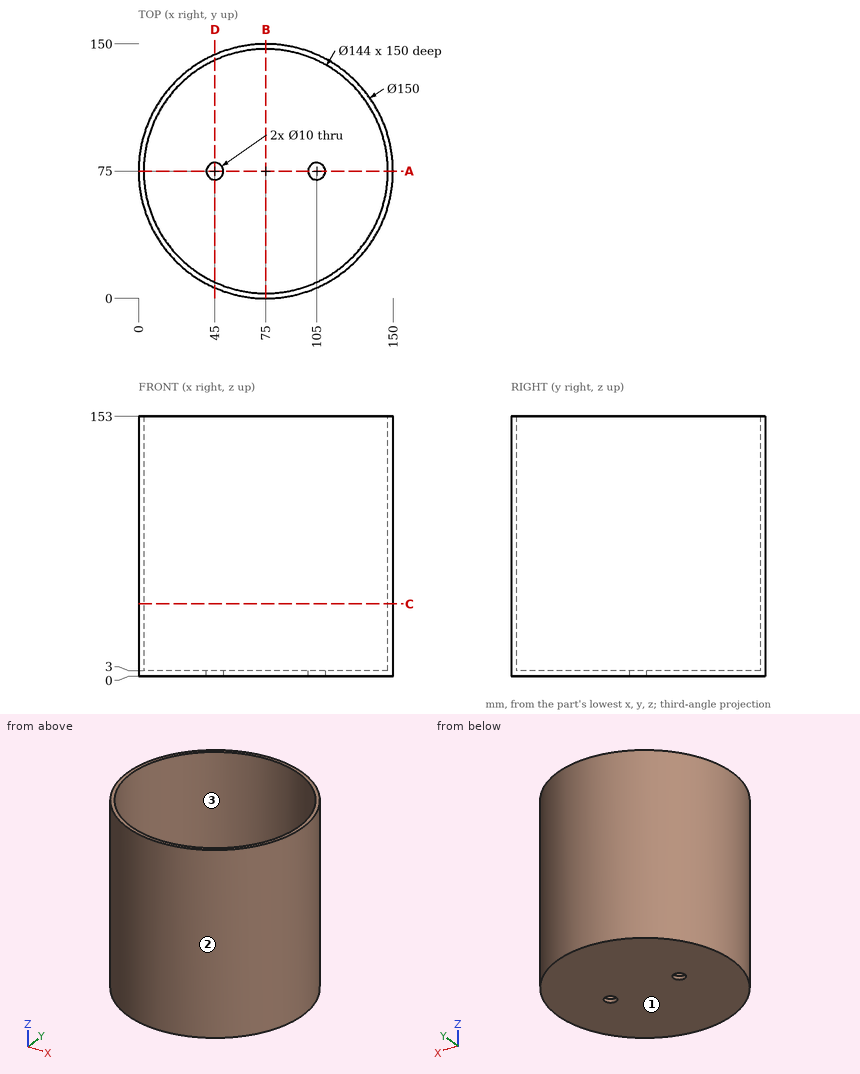
Can you work these out from the drawing? Everything is in mm from the part's minimum corner. Coordinates: 2 decimals unless noted, no trailing zeros. Loops run counter-clockwise (first coordinate to the right, second up) from the corner with the lowest first, then second, coordinate; pieces in that order, holes last.
1. Imagine slicing it at C-C, the plane z = 42.5. Please give me the cut outline in (x, y).
2. Imagine slicing it at A-A, the plane y = 75. Please give me the cut outline in (x, z), and give its area (3 significant figures).
3. For P1, Ø10, axis at x = 76.5, y = 112, coming from the +Z side; P2, Ø6, axis at y = 81.5, z = 90.5, coming from the +X side; P3, Ø2, axis at x = 17.5, z = 107, coming from the -Y side; P4, Ø6, axis at x = 105, y = 75, coming from the -Z side, each with a flat end and sliding along its axis, tell me the tip position at first contact or that it passes through.
4. I need wall thicknesses on L1, parallel to Y at x = 75, z = 40.5; L2, parallel to Z at x = 103, y = 15; L3, parallel to Y at x = 59.5, z = 117. Which ranges of each line are inside material? Lowest first, please.
5. Imagine slicing it at D-D, the plane x = 45. Please give me the cut outline in (y, z), and give its area (3 significant figures).
6. Imagine slicing it at B-B, the plane x = 75. Please give me the cut outline in (y, z).
7. If we mould it in two halves opening along X, with no side actions, what happens to the marked faces 1, 2 and 3? For each: pulls with the +X half, pulls with the -X half, needs draft (parallel to the pull), parting line crosses it, or undercut.
Taken from the geometry:
1. outline: circle Ø150 at (75, 75); hole circle Ø144 at (75, 75)
2. outline: (0, 0) - (40, 0) - (40, 3) - (3, 3) - (3, 153) - (0, 153) - close; (50, 0) - (100, 0) - (100, 3) - (50, 3) - close; (110, 0) - (150, 0) - (150, 153) - (147, 153) - (147, 3) - (110, 3) - close
2. area: 1,290 mm2
3. P1: stops at z = 3
3. P2: stops at x = 149.92
3. P3: stops at y = 25.68
3. P4: passes through
4. L1: y = 0 to 3, 147 to 150
4. L2: z = 0 to 3
4. L3: y = 1.62 to 4.69, 145.31 to 148.38
5. outline: (6.26, 0) - (70, 0) - (70, 3) - (9.55, 3) - (9.55, 153) - (6.26, 153) - close; (80, 0) - (143.74, 0) - (143.74, 153) - (140.45, 153) - (140.45, 3) - (80, 3) - close
5. area: 1,370 mm2
6. outline: (0, 0) - (150, 0) - (150, 153) - (147, 153) - (147, 3) - (3, 3) - (3, 153) - (0, 153) - close
7. face 1: needs draft
7. face 2: parting line crosses it
7. face 3: undercut
